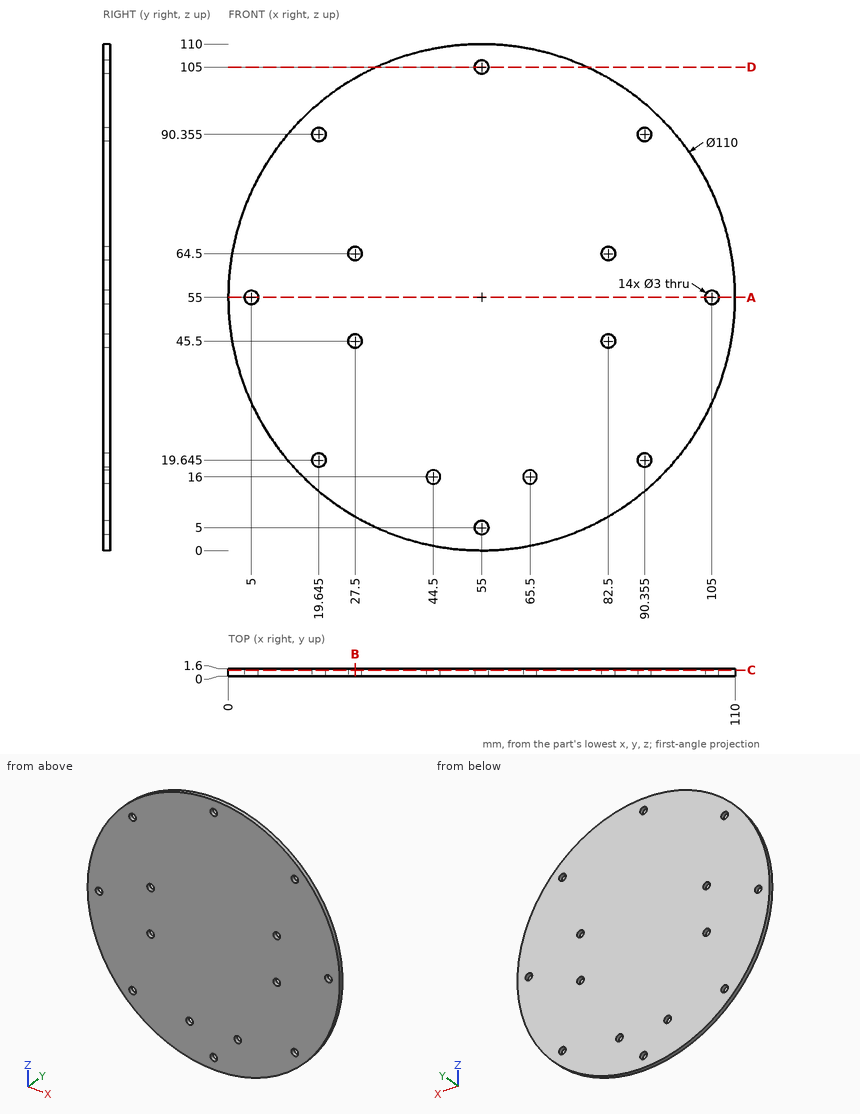
Here's the drawing with two shaded views (mm, measured from the low corner). I have some questions. Round coordinates to 2 decimals unless told otherwise and drop trailing zeros. Loops run counter-clockwise (first coordinate to the right, second up) from the corner with the lowest first, then second, coordinate; pieces in that order, holes last.
1. Suppose I cut it at C-C, the plane y = 1.3. Give the number of separate pieces and of enclosed holes in the cut face, and give its area (3 significant figures).
Answers:
separate pieces: 1
enclosed holes: 14
area: 9,400 mm2
2. If I drill on probe 1 along Z at (x, y) = (55, 0.8); probe 2 along Z at (x, y) = (19, 0.5); probe 3 along X at (y, z) = (1.15, 5) (1 decimal), over which ranges is the centre line in solid material (lowest first)?
Answers:
probe 1: z = 0 to 3.5, 6.5 to 103.5, 106.5 to 110
probe 2: z = 13.42 to 18.29, 21 to 89, 91.71 to 96.58
probe 3: x = 32.1 to 53.5, 56.5 to 77.9
3. Suppose I cut it at D-D, the plane z = 105. Please give me the cut outline in (x, y).
Answers:
outline: (32.09, 0) - (53.5, 0) - (53.5, 1.6) - (32.09, 1.6) - close; (56.5, 0) - (77.91, 0) - (77.91, 1.6) - (56.5, 1.6) - close
4. Suppose I cut it at A-A, the plane z = 55. Please give me the cut outline in (x, y).
Answers:
outline: (0, 0) - (3.5, 0) - (3.5, 1.6) - (0, 1.6) - close; (6.5, 0) - (103.5, 0) - (103.5, 1.6) - (6.5, 1.6) - close; (106.5, 0) - (110, 0) - (110, 1.6) - (106.5, 1.6) - close
5. Suppose I cut it at B-B, the plane x = 27.5. Please give me the cut outline in (y, z), and give its area (3 significant figures).
Answers:
outline: (0, 7.37) - (1.6, 7.37) - (1.6, 44) - (0, 44) - close; (0, 47) - (1.6, 47) - (1.6, 63) - (0, 63) - close; (0, 66) - (1.6, 66) - (1.6, 102.63) - (0, 102.63) - close
area: 143 mm2
